Input: part model. Units: mm. Frame: model coordinates. Face numbers are marked on the shaded views. Give positions to 0.01 mm unless a question says otherwise; leave off trailing zeros. Write each loop counter-clockwise with the first axis right and the second up, starting at its lowest first coordinate (ties: lowest second). Pieces come first, ordered by that corner, then holes. Notation, with made-up numbers: (69, 76.5) - (110, 76.5) arc R4 ccw to (110, 83.5) - close; hole circle Ø10 at (82.25, 84.5). An arc over 180 degrees is marked (long way). Use a Markdown table: item, result. Add a question column.
1. Section query C-C, the plane z = 10.75. Return loops of the section in (x, y), plus the area to 3 significant figures.
2. Section query B-B, the plane y = 3. Return loops of the section in (x, z), plus the area to 3 significant figures.
3. Mould query, pull axis X, two halves, no side actions, for the marked faces 1, 2, 3 and 4. Classes: released by +X, released by -X, zero draft, split by the parting line, or undercut.
4. Section query A-A, the plane z = 25. Return loops of the section in (x, y) (1 decimal), plus the area to 3 significant figures.
5. Material intervals for probe 1 along X at (y, z) = (1.5, 4); probe 2 along Z at (x, y) = (-27.25, -6); probe 3 along Y at (x, z) = (-24.5, 15.5), sorted ascending.
6. Pin query (flat end, axial travel): pin 1 (3 mm diameter, centred on y = -5.33, z = 4.953, fed in from -X); pin 2 (1.2 mm diameter, centred on x = -26.5, y = 3.5, fed in from +Z); pin 3 (2.5 mm diameter, centred on x = -27.3, y = -13.27, fed in from -Z). Return the tip coordinate at first contact, or that it passes through.
7. Section query D-D, the plane x = -28.5. Return loops of the section in (y, z), plus the area to 3 significant figures.
```python
from build123d import *

# Parameters (mm, degrees)
SKETCH028_R     = 1.75
SKETCH028_R_2   = 4.318
PAD017_DEPTH    = 6.35
SKETCH036_R     = 2
POCKET014_DEPTH = 6.35
SKETCH050_R     = 2.286
POCKET022_DEPTH = 4.318


with BuildPart() as part:
    # Sketch028 → Pad017 (new body)
    with BuildSketch(Plane.YZ):
        Polygon((12.3825, 0), (-12.3825, 0), (-12.3825, 29.464), (-1.4605, 29.464), (0, 29.0286659329), (1.4605, 29.464), (12.3825, 29.464), align=None)
        with Locations((0, 24.003)):
            Circle(SKETCH028_R, mode=Mode.SUBTRACT)
        with Locations((8.0645, 14.478)):
            Circle(SKETCH028_R, mode=Mode.SUBTRACT)
        with Locations((0, 4.953)):
            Circle(SKETCH028_R, mode=Mode.SUBTRACT)
        with Locations((-8.0645, 14.478)):
            Circle(SKETCH028_R, mode=Mode.SUBTRACT)
        with Locations((0, 14.478)):
            Circle(SKETCH028_R_2, mode=Mode.SUBTRACT)
    extrude(amount=-PAD017_DEPTH)

    # Sketch036 (on Face1 of Pad017) → Pocket014 (cut)
    with BuildSketch(Plane(origin=(0, 0, 29.464), x_dir=(0, -1, 0), z_dir=(0, 0, 1))):
        with Locations((-8.0310998827, -3.175)):
            Circle(SKETCH036_R)
        with Locations((8.0310998827, -3.175)):
            Circle(SKETCH036_R)
    extrude(amount=-POCKET014_DEPTH, mode=Mode.SUBTRACT)

    # Sketch050 (on Face8 of Pocket014) → Pocket022 (cut)
    with BuildSketch(Plane.YX):
        with Locations((-7.9375, -3.175)):
            Circle(SKETCH050_R)
        with Locations((7.9375, -3.175)):
            Circle(SKETCH050_R)
    extrude(amount=-POCKET022_DEPTH, mode=Mode.SUBTRACT)


with BuildPart() as part_1:
    # Body010 placement: moved
    add(part.part.moved(Location((-24.13, -5.33, 0))))


solid = part_1.part
```
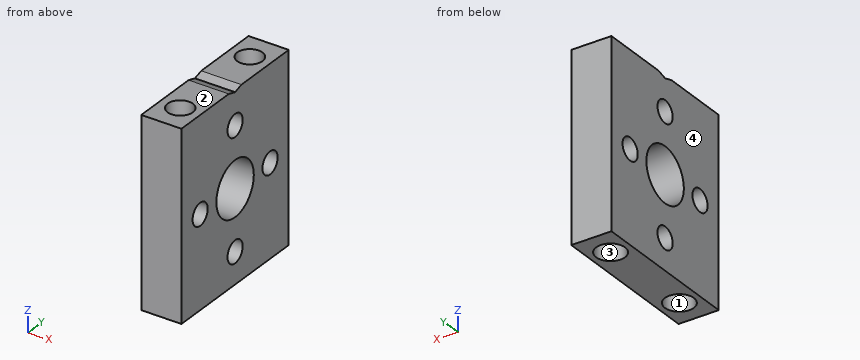
Result sheet:
| question | item | result |
|---|---|---|
| 1 | outline | (-30.48, -17.71) - (-24.13, -17.71) - (-24.13, -7.51) - (-30.48, -7.51) - close; (-30.48, -3.15) - (-24.13, -3.15) - (-24.13, 7.05) - (-30.48, 7.05) - close |
| 1 | area | 130 mm² |
| 2 | outline | (-30.48, 0) - (-29.56, 0) - (-29.56, 4.32) - (-25.05, 4.32) - (-25.05, 0) - (-24.13, 0) - (-24.13, 12.75) - (-30.48, 12.75) - close; (-30.48, 16.21) - (-24.13, 16.21) - (-24.13, 29.46) - (-25.33, 29.46) - (-25.33, 23.11) - (-29.28, 23.11) - (-29.28, 29.46) - (-30.48, 29.46) - close |
| 2 | area | 121 mm² |
| 3 | face 1 | undercut |
| 3 | face 2 | zero draft |
| 3 | face 3 | undercut |
| 3 | face 4 | released by -X |
| 4 | outline | (-30.5, -17.7) - (-24.1, -17.7) - (-24.1, -6.8) - (-30.5, -6.8) - close; (-30.5, -3.9) - (-24.1, -3.9) - (-24.1, 7.1) - (-30.5, 7.1) - close; hole circle Ø4 at (-27.3, -13.4); hole circle Ø4 at (-27.3, 2.7) |
| 4 | area | 114 mm² |
| 5 | probe 1 | x = -30.48 to -29.3, -25.31 to -24.13 |
| 5 | probe 2 | z = 0 to 3.34, 6.57 to 10.21, 18.74 to 22.39, 25.62 to 29.23 |
| 5 | probe 3 | y = -17.71 to -14.82, -11.97 to -9.53, -1.13 to 1.31, 4.16 to 7.05 |
| 6 | pin 1 | passes through |
| 6 | pin 2 | stops at z = 23.11 |
| 6 | pin 3 | stops at z = 4.32 |
| 7 | outline | (-17.71, 0) - (-15.22, 0) - (-15.22, 4.32) - (-11.32, 4.32) - (-11.32, 0) - (0.66, 0) - (0.66, 4.32) - (4.56, 4.32) - (4.56, 0) - (7.05, 0) - (7.05, 29.46) - (4.3, 29.46) - (4.3, 23.11) - (1.1, 23.11) - (1.1, 29.46) - (-3.87, 29.46) - (-5.33, 29.03) - (-6.79, 29.46) - (-11.76, 29.46) - (-11.76, 23.11) - (-14.96, 23.11) - (-14.96, 29.46) - (-17.71, 29.46) - close; hole circle Ø3.5 at (-13.39, 14.48); hole circle Ø8.64 at (-5.33, 14.48); hole circle Ø3.5 at (-5.33, 4.95); hole circle Ø3.5 at (-5.33, 24); hole circle Ø3.5 at (2.73, 14.48) |
| 7 | area | 558 mm² |
